from build123d import *

# Parameters (mm, degrees)
F1_DEPTH     = 5
F3_DEPTH     = 2
F4_R         = 2.5
F5_T1_DEPTH  = 27.4519311484
F5_T3_DEPTH  = 1.45667481
F5_T5_DEPTH  = 1.1206167057
F5_T7_DEPTH  = 31.3076734299
F5_T9_DEPTH  = 4.3560651868
F5_T11_DEPTH = 1.45667481
F5_T13_DEPTH = 4.3560651868
F5_T16_ANGLE = 24.1585538769
F5_T18_ANGLE = 65.8414461231
F5_T20_ANGLE = 35.4104549915
F5_T22_ANGLE = 65.8414461231
F5_T24_ANGLE = 54.5895450085
F5_T26_ANGLE = 24.1585538769
F5_T28_ANGLE = 54.5895450085
F5_T30_ANGLE = 35.4104549915


# Not quite as in the source:
# - a fillet or chamfer that OpenCascade refuses, or shapes differently, is made with other operations: its cross-section is extruded or revolved along the edge and cut away or added


with BuildPart() as f1:
    # F0 (on Top) → F1 (new body)
    with BuildSketch(Plane.XY):
        Polygon((18.75, 6.7059138706), (17.27244219, 10), (0, 10), (-17.27244219, 10), (-18.75, 6.7059138706), (-18.75, 4.2521861975), (-15.0160229505, -1), (0, -1), (15.0160229505, -1), (18.75, 4.2521861975), align=None)
        Polygon((14.5, 0), (0, 0), (-14.5, 0), (-17.75, 4.5714274394), (-17.75, 6.4919107255), (-16.625, 9), (0, 9), (16.625, 9), (17.75, 6.4919107255), (17.75, 4.5714274394), align=None, mode=Mode.SUBTRACT)
    extrude(amount=F1_DEPTH)



with BuildPart() as f1b:
    # F0 (on Top) → F1, piece 2 (new body)
    with BuildSketch(Plane.XY):
        Polygon((-15.4919761674, 7.25), (-16, 6.1174052217), (-16, 5.1300996126), (-13.5969598365, 1.75), (-13, 1.75), (-13, 7.25), align=None)
    extrude(amount=F1_DEPTH)


with BuildPart() as f1c:
    # F0 (on Top) → F1, piece 3 (new body)
    with BuildSketch(Plane.XY):
        Polygon((16, 6.1174052217), (15.4919761674, 7.25), (13, 7.25), (13, 1.75), (13.5969598365, 1.75), (16, 5.1300996126), align=None)
    extrude(amount=F1_DEPTH)


with BuildPart() as f1_1:
    add(f1.part)

    add(f1b.part)  # F3 merges F1b

    add(f1c.part)  # F3 merges F1c
    # F2 (on face) → F3 (join)
    with BuildSketch(Plane(origin=(0, 0, 0), x_dir=(1, 0, 0), z_dir=(0, 0, -1))):
        Polygon((-17.27244219, -10), (17.27244219, -10), (18.75, -6.7059138706), (18.75, -4.2521861975), (15.0160229505, 1), (-15.0160229505, 1), (-18.75, -4.2521861975), (-18.75, -6.7059138706), align=None)
    extrude(amount=F3_DEPTH)

    # F4
    f4_edges = [f1_1.edges().sort_by_distance(p)[0] for p in [
        (-18.75, 5.47905, -2),
        (-18.011221, 8.352957, -2),
        (0, 10, -2),
        (18.011221, 8.352957, -2),
        (18.75, 5.47905, -2),
        (16.883011, 1.626093, -2),
        (0, -1, -2),
        (-16.883011, 1.626093, -2),
        (-15.016023, -1, 1.5),
        (-18.75, 4.252186, 1.5),
        (-18.75, 6.705914, 1.5),
        (-17.272442, 10, 1.5),
        (15.016023, -1, 1.5),
        (18.75, 4.252186, 1.5),
        (17.272442, 10, 1.5),
        (18.75, 6.705914, 1.5),
    ]]
    fillet(f4_edges, radius=F4_R)

    # F5: fillet of radius 1 on 16 edges, made by hand

    # F5_s2 → F5_t1 (cut)
    with BuildSketch(Plane.YZ.offset(-13.7259655742)):
        with BuildLine():
            ThreePointArc((0, 5), (-0.7071067812, 4.7071067812), (-1, 4))
            Line((-1, 4), (-1, 5))
            Line((-1, 5), (0, 5))
        make_face()
    extrude(amount=F5_T1_DEPTH, mode=Mode.SUBTRACT)

    # F5_s4 → F5_t3 (cut)
    with BuildSketch(Plane(origin=(0.417485186, -0.9307467709, 0), x_dir=(0, 0, 1), z_dir=(-0.4092631251, 0.9124164041, 0))):
        with BuildLine():
            ThreePointArc((4, 19.8522908438), (4.7071067812, 19.5593976249), (5, 18.8522908438))
            Line((5, 18.8522908438), (5, 19.8522908438))
            Line((5, 19.8522908438), (4, 19.8522908438))
        make_face()
    extrude(amount=F5_T3_DEPTH, mode=Mode.SUBTRACT)

    # F5_s6 → F5_t5 (cut)
    with BuildSketch(Plane.XZ.offset(-6.1709060079)):
        with BuildLine():
            ThreePointArc((17.75, 5), (18.4571067812, 4.7071067812), (18.75, 4))
            Line((18.75, 4), (18.75, 5))
            Line((18.75, 5), (17.75, 5))
        make_face()
        with BuildLine():
            ThreePointArc((-17.75, 5), (-18.4571067812, 4.7071067812), (-18.75, 4))
            Line((-18.75, 4), (-18.75, 5))
            Line((-18.75, 5), (-17.75, 5))
        make_face()
    extrude(amount=F5_T5_DEPTH, mode=Mode.SUBTRACT)

    # F5_s8 → F5_t7 (cut)
    with BuildSketch(Plane.YZ.offset(-15.6538367149)):
        with BuildLine():
            ThreePointArc((9, 5), (9.7071067812, 4.7071067812), (10, 4))
            Line((10, 4), (10, 5))
            Line((10, 5), (9, 5))
        make_face()
    extrude(amount=F5_T7_DEPTH, mode=Mode.SUBTRACT)

    # F5_s10 → F5_t9 (cut)
    with BuildSketch(Plane(origin=(5.3167143619, 7.4784535142, 0), x_dir=(0, 0, 1), z_dir=(0.5794299023, 0.8150220784, 0))):
        with BuildLine():
            ThreePointArc((5, 11.8178201367), (4.7071067812, 12.5249269179), (4, 12.8178201367))
            Line((4, 12.8178201367), (5, 12.8178201367))
            Line((5, 12.8178201367), (5, 11.8178201367))
        make_face()
    extrude(amount=F5_T9_DEPTH, mode=Mode.SUBTRACT)

    # F5_s12 → F5_t11 (cut)
    with BuildSketch(Plane(origin=(0.1786780991, 0.3983472212, 0), x_dir=(0, 0, 1), z_dir=(-0.4092631251, -0.9124164041, 0))):
        with BuildLine():
            ThreePointArc((5, 18.8522908438), (4.7071067812, 19.5593976249), (4, 19.8522908438))
            Line((4, 19.8522908438), (5, 19.8522908438))
            Line((5, 19.8522908438), (5, 18.8522908438))
        make_face()
    extrude(amount=F5_T11_DEPTH, mode=Mode.SUBTRACT)

    # F5_s14 → F5_t13 (cut)
    with BuildSketch(Plane(origin=(-7.8407487877, 11.0287428164, 0), x_dir=(0, 0, 1), z_dir=(0.5794299023, -0.8150220784, 0))):
        with BuildLine():
            ThreePointArc((5, 11.8178201367), (4.7071067812, 12.5249269179), (4, 12.8178201367))
            Line((4, 12.8178201367), (5, 12.8178201367))
            Line((5, 12.8178201367), (5, 11.8178201367))
        make_face()
    extrude(amount=F5_T13_DEPTH, mode=Mode.SUBTRACT)

    # F5_s15 → F5_t16 (revolve, cut)
    with BuildSketch(Plane(origin=(0.417485186, -0.9307467709, 0), x_dir=(0, 0, 1), z_dir=(-0.4092631251, 0.9124164041, 0))):
        with BuildLine():
            ThreePointArc((5, 18.8522908438), (4.7071067812, 19.5593976249), (4, 19.8522908438))
            Line((4, 19.8522908438), (5, 19.8522908438))
            Line((5, 19.8522908438), (5, 18.8522908438))
        make_face()
    revolve(axis=Axis((16.25, 6.1709060079, 5), (0, 0, -1)), revolution_arc=F5_T16_ANGLE, mode=Mode.SUBTRACT)

    # F5_s17 → F5_t18 (revolve, cut)
    with BuildSketch(Plane(origin=(-0.1786780991, 0.3983472212, 0), x_dir=(0, 0, 1), z_dir=(0.4092631251, -0.9124164041, 0))):
        with BuildLine():
            ThreePointArc((5, -18.8522908438), (4.7071067812, -19.5593976249), (4, -19.8522908438))
            Line((4, -19.8522908438), (5, -19.8522908438))
            Line((5, -19.8522908438), (5, -18.8522908438))
        make_face()
    revolve(axis=Axis((15.6538367149, 7.5, 5), (0, 0, 1)), revolution_arc=F5_T18_ANGLE, mode=Mode.SUBTRACT)

    # F5_s19 → F5_t20 (revolve, cut)
    with BuildSketch(Plane.XZ.offset(-5.0502893022)):
        with BuildLine():
            ThreePointArc((17.75, 5), (18.4571067812, 4.7071067812), (18.75, 4))
            Line((18.75, 4), (18.75, 5))
            Line((18.75, 5), (17.75, 5))
        make_face()
    revolve(axis=Axis((16.25, 5.0502893022, 5), (0, 0, -1)), revolution_arc=F5_T20_ANGLE, mode=Mode.SUBTRACT)

    # F5_s21 → F5_t22 (revolve, cut)
    with BuildSketch(Plane.YZ.offset(-15.6538367149)):
        with BuildLine():
            ThreePointArc((9, 5), (9.7071067812, 4.7071067812), (10, 4))
            Line((10, 4), (10, 5))
            Line((10, 5), (9, 5))
        make_face()
    revolve(axis=Axis((-15.6538367149, 7.5, 5), (0, 0, 1)), revolution_arc=F5_T22_ANGLE, mode=Mode.SUBTRACT)

    # F5_s23 → F5_t24 (revolve, cut)
    with BuildSketch(Plane(origin=(5.3167143619, 7.4784535142, 0), x_dir=(0, 0, 1), z_dir=(0.5794299023, 0.8150220784, 0))):
        with BuildLine():
            ThreePointArc((5, 11.8178201367), (4.7071067812, 12.5249269179), (4, 12.8178201367))
            Line((4, 12.8178201367), (5, 12.8178201367))
            Line((5, 12.8178201367), (5, 11.8178201367))
        make_face()
    revolve(axis=Axis((13.7259655742, 1.5, 5), (0, 0, -1)), revolution_arc=F5_T24_ANGLE, mode=Mode.SUBTRACT)

    # F5_s25 → F5_t26 (revolve, cut)
    with BuildSketch(Plane(origin=(-0.417485186, -0.9307467709, 0), x_dir=(0, 0, 1), z_dir=(0.4092631251, 0.9124164041, 0))):
        with BuildLine():
            ThreePointArc((5, -18.8522908438), (4.7071067812, -19.5593976249), (4, -19.8522908438))
            Line((4, -19.8522908438), (5, -19.8522908438))
            Line((5, -19.8522908438), (5, -18.8522908438))
        make_face()
    revolve(axis=Axis((-16.25, 6.1709060079, 5), (0, 0, 1)), revolution_arc=F5_T26_ANGLE, mode=Mode.SUBTRACT)

    # F5_s27 → F5_t28 (revolve, cut)
    with BuildSketch(Plane(origin=(-5.3167143619, 7.4784535142, 0), x_dir=(0, 0, 1), z_dir=(-0.5794299023, 0.8150220784, 0))):
        with BuildLine():
            ThreePointArc((5, -11.8178201367), (4.7071067812, -12.5249269179), (4, -12.8178201367))
            Line((4, -12.8178201367), (5, -12.8178201367))
            Line((5, -12.8178201367), (5, -11.8178201367))
        make_face()
    revolve(axis=Axis((-13.7259655742, 1.5, 5), (0, 0, 1)), revolution_arc=F5_T28_ANGLE, mode=Mode.SUBTRACT)

    # F5_s29 → F5_t30 (revolve, cut)
    with BuildSketch(Plane.XZ.offset(-5.0502893022)):
        with BuildLine():
            ThreePointArc((-17.75, 5), (-18.4571067812, 4.7071067812), (-18.75, 4))
            Line((-18.75, 4), (-18.75, 5))
            Line((-18.75, 5), (-17.75, 5))
        make_face()
    revolve(axis=Axis((-16.25, 5.0502893022, 5), (0, 0, 1)), revolution_arc=F5_T30_ANGLE, mode=Mode.SUBTRACT)


solid = f1_1.part
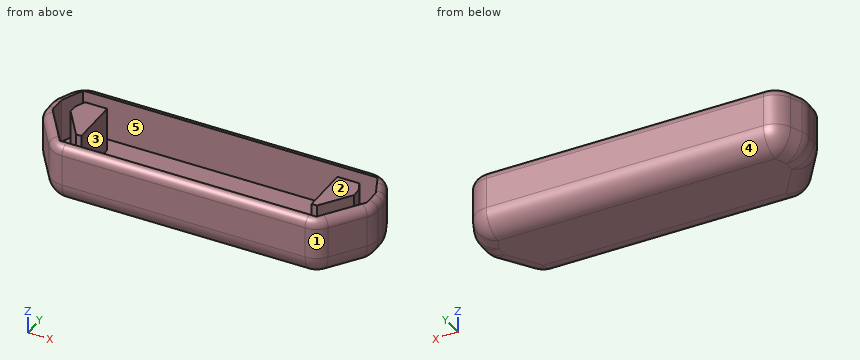
Build history of the part. All positions in model axes, mm. Face numbers are marked on the shaded views. A direction names the side the tool comes from. Give positions to 0.01 mm unless a question says otherwise; leave off trailing zeros. Write each loop counter-clockwise with the first axis right and the second up, starting at its lowest first coordinate (ties: lowest second). Pieces come first, ordered by that corner, then holes. Notation, with made-up numbers: (5.25, 69) - (19.25, 69) arc R23 ccw to (19.25, 79) - close; hole circle Ø1 at (66.25, 50.5). An arc over 180 degrees is marked (long way). Use one line per item in the form item = value. Start each with the question number.
1. Drop a flat-ended pin along its axis: pin 1 Ø2 at (x, y) = (-5, 2.5) entering from +Z. Give the stop position or say it passes through.
2. Band-saw the part on B-B on x = -8.5. Write the cut outline in (y, z).
3. Band-saw the part on C-C on z = -1.25. Write the cut outline in (x, y), plus the area to 3 significant figures.
4. Two-plate mould, pull along X, no slides. Class the marked faces 1, 2 and 3: released by +X, released by -X, zero draft, split by the parting line, or undercut.
5. Band-saw the part on A-A on z = 3. Count the separate pieces of the cut face and the enclosed holes in it, plus the area to 3 significant figures.
6. Probe line 1 (X direction, y = 3, z = 3.5); line 2 (Y direction, x = -10, z = 2.5); line 3 (X direction, y = 4, z = 4.75). List the from-to ranges inside material, lowest first. Write a range as [from, to].
7. 3-axis set-ups, long thin cutter, end or side, ignore diameter. For the marked faces 4 and 5: which of +Z, -Z, +X, -X, +Y, -Y reach the whole face in a straight line?
Conclusion:
q1.pin_1 = 0
q2.outline = (-1, 0.5) arc R2.5 ccw to (1.5, -2) - (7.5, -2) arc R2.5 ccw to (10, 0.5) - (10, 4) arc R1 ccw to (9, 5) - (9, 0) - (0, 0) - (0, 5) arc R1 ccw to (-1, 4) - close
q3.outline = (-18.04, 5.05) arc R1.79 ccw to (-17.71, 4.02) - (-15.18, 0.47) arc R1.79 ccw to (-13.73, -0.29) - (13.73, -0.29) arc R1.79 ccw to (15.18, 0.47) - (17.71, 4.02) arc R1.79 ccw to (18.04, 5.05) - (18.04, 6.17) arc R1.79 ccw to (17.88, 6.9) - (17.28, 8.23) arc R1.79 ccw to (15.65, 9.29) - (-15.65, 9.29) arc R1.79 ccw to (-17.28, 8.23) - (-17.88, 6.9) arc R1.79 ccw to (-18.04, 6.17) - close
q3.area = 325 mm²
q4.face_1 = released by +X
q4.face_2 = zero draft
q4.face_3 = undercut
q5.separate_pieces = 3
q5.enclosed_holes = 1
q5.area = 109 mm²
q6.line_1 = [-17.86, -16.63], [-14.49, -13], [13, 14.49], [16.63, 17.86]
q6.line_2 = [-1, 0], [9, 10]
q6.line_3 = [-18.14, -17.34], [-15.2, -13], [13, 15.2], [17.34, 18.14]
q7.face_4 = -Z, +X, -X, +Y
q7.face_5 = +Z
